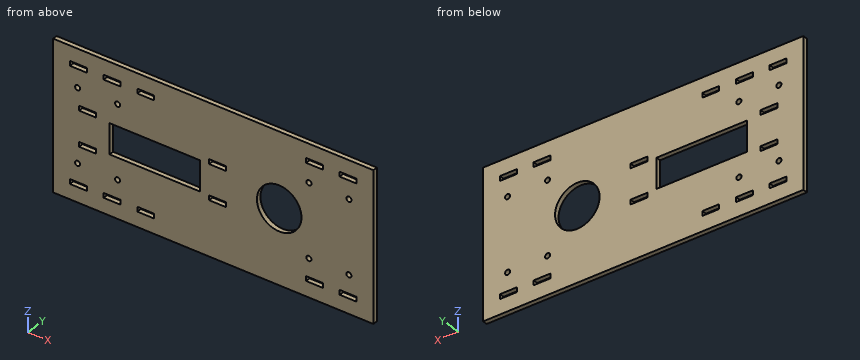
```python
from build123d import *

# Parameters (mm, degrees)
SKETCH1_W               = 215.9
SKETCH1_H               = 100
BOSS_EXTRUDE1_DEPTH     = 3.175
SKETCH3_W               = 11.35
SKETCH3_H               = 3.175
CUT_EXTRUDE2_DEPTH      = 3.175
SKETCH4_W               = 11.35
SKETCH4_H               = 3.175
CUT_EXTRUDE3_DEPTH      = 3.175
SKETCH5_W               = 60.96
SKETCH5_H               = 20.32
CUT_EXTRUDE4_DEPTH      = 1
CUT_EXTRUDE4_DEPTH_BACK = 3.175
SKETCH6_R               = 1.7145
CUT_EXTRUDE5_DEPTH      = 3.175
SKETCH7_R               = 15
CUT_EXTRUDE6_DEPTH      = 3.175
SKETCH8_W               = 11.35
SKETCH8_H               = 3.175
CUT_EXTRUDE7_DEPTH      = 3.175


with BuildPart() as part:
    # Sketch1 → Boss-Extrude1 (new body)
    with BuildSketch(Plane(origin=(0, 0, 0), x_dir=(1, 0, 0), z_dir=(0, 1, 0))):
        with Locations((-1.255776173, 17.463898917)):
            Rectangle(SKETCH1_W, SKETCH1_H)
    extrude(amount=BOSS_EXTRUDE1_DEPTH)

    # Sketch3 → Cut-Extrude2 (cut)
    with BuildSketch(Plane(origin=(0, 3.175, 0), x_dir=(1, 0, 0), z_dir=(0, 1, 0))):
        with Locations((-92.180776173, 55.876398917)):
            Rectangle(SKETCH3_W, SKETCH3_H)
        with Locations((-46.780776173, 55.876398917)):
            Rectangle(SKETCH3_W, SKETCH3_H)
        with Locations((-69.480776173, 55.876398917)):
            Rectangle(SKETCH3_W, SKETCH3_H)
        with Locations((66.969233827, 55.876398917)):
            Rectangle(SKETCH3_W, SKETCH3_H)
        with Locations((89.669223827, 55.876398917)):
            Rectangle(SKETCH3_W, SKETCH3_H)
    extrude(amount=-CUT_EXTRUDE2_DEPTH, mode=Mode.SUBTRACT)

    # Sketch4 → Cut-Extrude3 (cut)
    with BuildSketch(Plane(origin=(0, 3.175, 0), x_dir=(1, 0, 0), z_dir=(0, 1, 0))):
        with Locations((-92.180776173, -20.948601083)):
            Rectangle(SKETCH4_W, SKETCH4_H)
        with Locations((-69.480776173, -20.948601083)):
            Rectangle(SKETCH4_W, SKETCH4_H)
        with Locations((-46.780776173, -20.948601083)):
            Rectangle(SKETCH4_W, SKETCH4_H)
        with Locations((66.969233827, -20.948601083)):
            Rectangle(SKETCH4_W, SKETCH4_H)
        with Locations((89.669223827, -20.948601083)):
            Rectangle(SKETCH4_W, SKETCH4_H)
    extrude(amount=-CUT_EXTRUDE3_DEPTH, mode=Mode.SUBTRACT)

    # Sketch5 → Cut-Extrude4 (cut, two sides)
    with BuildSketch(Plane(origin=(0, 3.175, 0), x_dir=(1, 0, 0), z_dir=(0, 1, 0))) as cut_extrude4_sk:
        with Locations((-40.625776173, 17.503898917)):
            Rectangle(SKETCH5_W, SKETCH5_H)
    extrude(amount=CUT_EXTRUDE4_DEPTH, mode=Mode.SUBTRACT)
    extrude(cut_extrude4_sk.sketch, amount=-CUT_EXTRUDE4_DEPTH_BACK, mode=Mode.SUBTRACT)

    # Sketch6 → Cut-Extrude5 (cut)
    with BuildSketch(Plane(origin=(0, 3.175, 0), x_dir=(1, 0, 0), z_dir=(0, 1, 0))):
        with Locations((-92.695776173, 42.063898917)):
            Circle(SKETCH6_R)
        with Locations((-65.746376173, 42.063898917)):
            Circle(SKETCH6_R)
        with Locations((-92.695776173, -7.136101083)):
            Circle(SKETCH6_R)
        with Locations((-65.746376173, -7.136101083)):
            Circle(SKETCH6_R)
        with Locations((63.234823827, 42.063898917)):
            Circle(SKETCH6_R)
        with Locations((90.184223827, 42.063898917)):
            Circle(SKETCH6_R)
        with Locations((63.234823827, -7.136101083)):
            Circle(SKETCH6_R)
        with Locations((90.184223827, -7.136101083)):
            Circle(SKETCH6_R)
    extrude(amount=-CUT_EXTRUDE5_DEPTH, mode=Mode.SUBTRACT)

    # Sketch7 → Cut-Extrude6 (cut)
    with BuildSketch(Plane(origin=(0, 3.175, 0), x_dir=(1, 0, 0), z_dir=(0, 1, 0))):
        with Locations((43.194223827, 17.463898917)):
            Circle(SKETCH7_R)
    extrude(amount=-CUT_EXTRUDE6_DEPTH, mode=Mode.SUBTRACT)

    # Sketch8 → Cut-Extrude7 (cut)
    with BuildSketch(Plane(origin=(0, 3.175, 0), x_dir=(1, 0, 0), z_dir=(0, 1, 0))):
        with Locations((-86.004776173, 5.756398917)):
            Rectangle(SKETCH8_W, SKETCH8_H)
        with Locations((-86.004776173, 29.251398917)):
            Rectangle(SKETCH8_W, SKETCH8_H)
        with Locations((1.705223827, 5.756398917)):
            Rectangle(SKETCH8_W, SKETCH8_H)
        with Locations((1.705223827, 29.251398917)):
            Rectangle(SKETCH8_W, SKETCH8_H)
    extrude(amount=-CUT_EXTRUDE7_DEPTH, mode=Mode.SUBTRACT)


solid = part.part
```
Source: CAD feature listing. Evaluate the final solid. Frame: model axes, mm. Give positions to 0.01 mm unless a question says otherwise; leave off trailing zeros. Loops run counter-clockwise (first coordinate to the right, second up) from the corner with the lowest first, then second, coordinate; pieces in that order, holes last. Notation, with made-up numbers: (3, 40) - (10, 40) arc R28 ccw to (10, 64) - close; hole circle Ø9 at (-20, -22.5). An arc over 180 degrees is marked (long way). Use CSV: the item, a comma, the result in double quotes.
1) Line query: line 1 (X direction, y = 1.5, z = 7.5); line 2 (Z direction, x = -95.5, y = 0.4); line 3 (Z direction, x = -41, y = 2). Output: solid intervals per line, ascending.
Worked out:
line 1,"x = -109.21 to -94.37, -91.02 to -67.42, -64.07 to 61.56, 64.91 to 88.51, 91.86 to 106.69"
line 2,"z = -67.46 to -57.46, -54.29 to 19.36, 22.54 to 32.54"
line 3,"z = -67.46 to -27.66, -7.34 to 32.54"
2) Cut plane A-A (x = -15). Output: boundary loops of the cut face in (y, z) (3 decimals), and give its area (3 significant figures).
Worked out:
outline,"(0, -67.464) - (3.175, -67.464) - (3.175, -27.664) - (0, -27.664) - close; (0, -7.344) - (3.175, -7.344) - (3.175, 32.536) - (0, 32.536) - close"
area,"253 mm^2"
3) Cut plane B-B (z = -20.5). Output: boundary loops of the cut face in (x, y) (3 decimals), and give its area (3 significant figures).
Worked out:
outline,"(-109.206, 0) - (-71.106, 0) - (-71.106, 3.175) - (-109.206, 3.175) - close; (-10.146, 0) - (28.505, 0) - (28.505, 3.175) - (-10.146, 3.175) - close; (57.884, 0) - (106.694, 0) - (106.694, 3.175) - (57.884, 3.175) - close"
area,"399 mm^2"
4) Cut plane D-D (y = 1.9). Count the separate pieces of the cut face and the enclosed holes in it, and give its area (3 significant figures).
Worked out:
separate pieces,"1"
enclosed holes,"24"
area,"19,100 mm^2"
5) Cut plane C-C (x = 55.5). Output: boundary loops of the cut face in (y, z) (3 decimals).
Worked out:
outline,"(0, -67.464) - (3.175, -67.464) - (3.175, -26.041) - (0, -26.041) - close; (0, -8.887) - (3.175, -8.887) - (3.175, 32.536) - (0, 32.536) - close"
